Build history of the part. All positions in model axes, mm. Face numbers are marked on the shaded views. A direction names the side the tool comes from. Round coordinates to 2 decimals unless told otherwise and drop trailing zeros. Loops run counter-clockwise (first coordinate to the right, second up) from the corner with the lowest first, then second, coordinate; pieces in that order, holes last. Notation, with made-up numbers: (86, 89.5) -> (139, 89.5) arc R30 cw to (139, 123.5) -> close; hole circle Ø11 at (-11.75, 78.5). An arc over 180 degrees is marked (long way). Put each result on its own line as item: value. Start each with the question number.
Item 1: Drill centre lines: probe 1 along Y at (x, z) = (14, 49.5); probe 2 along Z at (x, y) = (23.5, -10); probe 3 along Z at (x, y) = (39.5, 0.5). Where is each one in solid material? Low to high. Write a range as [from, to].
Item 2: Cut at A-A, the plane x = 6. List the corners of the cut face in (y, z).
Item 3: Flat gauge pins, fed straight in: pin 1 Ø8 at (x, z) = (43.5, 38.5) entering from -Y; pin 2 Ø10 at (x, z) = (21.5, 45.5) entering from -Y; pin 3 Ø24.5 at (x, z) = (26, 63.5) entering from -Y. Where does each tip first touch, or does it go through?
Item 4: Cut at B-B, the plane y = -24.5. List the corners of the cut face in (x, z).
Item 5: Cut at C-C, the plane y = -16. List the corners of the cut face in (x, z), plus the area to 3 significant figures.
Item 6: Tool access for the marked faces 1 and 2: list every direction of +Z, -Z, +X, -X, +Y, -Y with a clear straight run to the whole face (end or side of a thin tool).
```python
from build123d import *

# Parameters (mm, degrees)
F1_DEPTH    = 50
F2_T1_DEPTH = 50
F2_T3_DEPTH = 75
F2_T5_DEPTH = 63.9698798509


# Not quite as in the source:
# - a fillet or chamfer that OpenCascade refuses, or shapes differently, is made with other operations: its cross-section is extruded or revolved along the edge and cut away or added


with BuildPart() as f1:
    # F0 (on Right) → F1 (new body)
    with BuildSketch(Plane.YZ):
        Polygon((-32.5, 24.4166636232), (-32.5, -50.5833363768), (7.5, -50.5833363768), (7.5, 74.4166636232), (0, 74.4166636232), (0, 44.4166636232), align=None)
    extrude(amount=F1_DEPTH)

    # F2: fillet of radius 5 on 4 edges, made by hand

    # F2_s2 → F2_t1 (join)
    with BuildSketch(Plane.YZ):
        with BuildLine():
            ThreePointArc((-2.3795128717, 42.9523480098), (-0.6352299235, 44.7716270515), (0, 47.2106395933))
            Line((0, 47.2106395933), (0, 44.4166636232))
            Line((0, 44.4166636232), (-2.3795128717, 42.9523480098))
        make_face()
    extrude(amount=F2_T1_DEPTH)

    # F2_s4 → F2_t3 (cut)
    with BuildSketch(Plane.YZ.offset(-12.5)):
        with BuildLine():
            ThreePointArc((5, 74.4166636232), (1.4644660941, 72.9521975291), (0, 69.4166636232))
            Line((0, 69.4166636232), (0, 74.4166636232))
            Line((0, 74.4166636232), (5, 74.4166636232))
        make_face()
        with BuildLine():
            ThreePointArc((7.5, 69.4166636232), (6.0355339059, 72.9521975291), (2.5, 74.4166636232))
            Line((2.5, 74.4166636232), (7.5, 74.4166636232))
            Line((7.5, 74.4166636232), (7.5, 69.4166636232))
        make_face()
    extrude(amount=F2_T3_DEPTH, mode=Mode.SUBTRACT)

    # F2_s6 → F2_t5 (cut)
    with BuildSketch(Plane.YZ.offset(-6.9849399255)):
        with BuildLine():
            ThreePointArc((-30.1204871283, 25.8809792365), (-31.8647700765, 24.0617001948), (-32.5, 21.622687653))
            Line((-32.5, 21.622687653), (-32.5, 24.4166636232))
            Line((-32.5, 24.4166636232), (-30.1204871283, 25.8809792365))
        make_face()
    extrude(amount=F2_T5_DEPTH, mode=Mode.SUBTRACT)


solid = f1.part
```
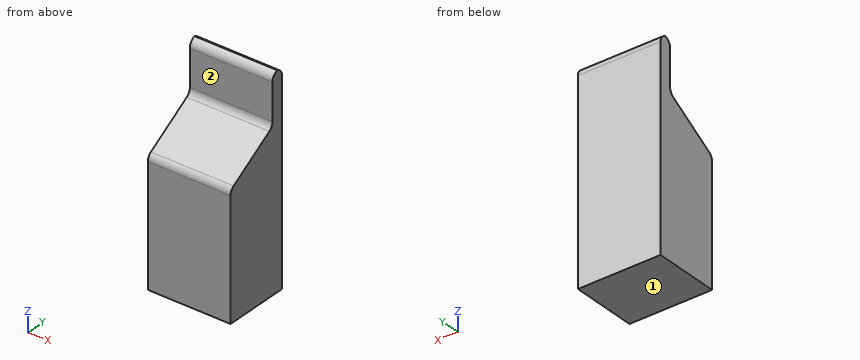
Reply:
1. probe 1: y = [0, 7.5]
1. probe 2: z = [-50.58, 38.26]
1. probe 3: z = [-50.58, 71.6]
2. outline: (-32.5, -50.58) -> (7.5, -50.58) -> (7.5, 69.42) arc R5 ccw to (3.75, 74.26) arc R5 ccw to (0, 69.42) -> (0, 47.21) arc R5 cw to (-2.38, 42.95) -> (-30.12, 25.88) arc R5 ccw to (-32.5, 21.62) -> close
3. pin 1: stops at y = -16.11
3. pin 2: stops at y = -6.36
3. pin 3: stops at y = 0
4. outline: (0, -50.58) -> (50, -50.58) -> (50, 29.34) -> (0, 29.34) -> close
5. outline: (0, -50.58) -> (50, -50.58) -> (50, 34.57) -> (0, 34.57) -> close
5. area: 4,260 mm^2
6. face 1: -Z, +X, -X, +Y, -Y
6. face 2: +Z, +X, -X, -Y
